from build123d import *

# Parameters (mm, degrees)
SKETCH_1_W             = 28
SKETCH_1_H             = 160
SKETCH_1_R             = 6
SKETCH_1_R_2           = 1.35
SM_BASE_FLANGE_1_DEPTH = 3
OTHER_START            = -14
OTHER_1_DEPTH          = 28
OTHER_1_2_DEPTH        = 28
SKETCH_7_R             = 1.35
CUT_EXTRUDE_1_DEPTH    = 81.582164958


# Read off the part's stored shape, not the designer's step: 绘制的折弯1
# Sheet-metal steps are written as plain solids
with BuildPart() as part:
    # Sketch 1 → 基体-法兰1 (new body)
    with BuildSketch(Plane(origin=(0, 0, 0), x_dir=(1, 0, 0), z_dir=(0, 1, 0))):
        Rectangle(SKETCH_1_W, SKETCH_1_H)
        with Locations(Location((0, 0, 0), (0, 0, 270))):
            Circle(SKETCH_1_R, mode=Mode.SUBTRACT)
        with Locations(Location((0, 11, 0), (0, 0, 270))):
            Circle(SKETCH_1_R_2, mode=Mode.SUBTRACT)
        with Locations(Location((7.778174593, 7.778174593, 0), (0, 0, 270))):
            Circle(SKETCH_1_R_2, mode=Mode.SUBTRACT)
        with Locations(Location((11, 0, 0), (0, 0, 270))):
            Circle(SKETCH_1_R_2, mode=Mode.SUBTRACT)
        with Locations(Location((7.778174593, -7.778174593, 0), (0, 0, 270))):
            Circle(SKETCH_1_R_2, mode=Mode.SUBTRACT)
        with Locations(Location((0, -11, 0), (0, 0, 270))):
            Circle(SKETCH_1_R_2, mode=Mode.SUBTRACT)
        with Locations(Location((-7.778174593, -7.778174593, 0), (0, 0, 270))):
            Circle(SKETCH_1_R_2, mode=Mode.SUBTRACT)
        with Locations(Location((-11, 0, 0), (0, 0, 270))):
            Circle(SKETCH_1_R_2, mode=Mode.SUBTRACT)
        with Locations(Location((-7.778174593, 7.778174593, 0), (0, 0, 270))):
            Circle(SKETCH_1_R_2, mode=Mode.SUBTRACT)
    extrude(amount=-SM_BASE_FLANGE_1_DEPTH)

    # Other 1 outline → Other 1 (cut)
    with BuildSketch(Plane.YZ.offset(OTHER_START)):
        with BuildLine():
            ThreePointArc((0, -31.146677222), (-2.154295979, -29.850867001), (-3, -27.4834))
            Line((-3, -27.4834), (-3, -80))
            Line((-3, -80), (0, -80))
            Line((0, -80), (0, -31.146677222))
        make_face()
        with BuildLine():
            Line((-3, 80), (-3, 22.7634))
            ThreePointArc((-3, 22.7634), (-2.154295979, 25.130867001), (0, 26.426677222))
            Line((0, 26.426677222), (0, 80))
            Line((0, 80), (-3, 80))
        make_face()
    extrude(amount=OTHER_1_DEPTH, mode=Mode.SUBTRACT)

    # Other 1 2 outline → Other 1 2 (add)
    with BuildSketch(Plane.YZ.offset(OTHER_START)):
        with BuildLine():
            Line((0, -27.4834), (0, -31.146677222))
            ThreePointArc((0, -31.146677222), (0.36647982, -31.201624121), (0.7366, -31.22))
            Line((0.7366, -31.22), (49.739956935, -31.22))
            Line((49.739956935, -31.22), (49.739956935, -28.22))
            Line((49.739956935, -28.22), (0.7366, -28.22))
            ThreePointArc((0.7366, -28.22), (0.215745145, -28.004254855), (0, -27.4834))
        make_face()
        with BuildLine():
            ThreePointArc((0.7366, 26.5), (0.36647982, 26.481624121), (0, 26.426677222))
            Line((0, 26.426677222), (0, 22.7634))
            ThreePointArc((0, 22.7634), (0.215745145, 23.284254855), (0.7366, 23.5))
            Line((0.7366, 23.5), (54.459956935, 23.5))
            Line((54.459956935, 23.5), (54.459956935, 26.5))
            Line((54.459956935, 26.5), (0.7366, 26.5))
        make_face()
    extrude(amount=OTHER_1_2_DEPTH)

    # 草图7 → 切除-拉伸1 (cut, through all)
    with BuildSketch(Plane(origin=(0, 0, -31.22), x_dir=(-1, 0, 0), z_dir=(0, 0, -1))):
        with Locations(Location((11, 32, 0), (0, 0, 90))):
            Circle(SKETCH_7_R)
        with Locations(Location((7.778174593, 24.221825407, 0), (0, 0, 90))):
            Circle(SKETCH_7_R)
        with Locations(Location((0, 21, 0), (0, 0, 90))):
            Circle(SKETCH_7_R)
        with Locations(Location((-7.778174593, 24.221825407, 0), (0, 0, 90))):
            Circle(SKETCH_7_R)
        with Locations(Location((-11, 32, 0), (0, 0, 90))):
            Circle(SKETCH_7_R)
        with BuildLine():
            Line((-14, 32), (-32.703539992, 32))
            Line((-32.703539992, 32), (-28.620805063, 56.964772816))
            Line((-28.620805063, 56.964772816), (24.538070134, 56.964772816))
            Line((24.538070134, 56.964772816), (24.538070134, 32))
            Line((24.538070134, 32), (14, 32))
            Line((14, 32), (14, 35.400052641))
            Line((14, 35.400052641), (6, 35.400052641))
            Line((6, 35.400052641), (6, 32))
            ThreePointArc((6, 32), (0, 26), (-6, 32))
            Line((-6, 32), (-6, 35.400052641))
            Line((-6, 35.400052641), (-14, 35.400052641))
            Line((-14, 35.400052641), (-14, 32))
        make_face()
    extrude(amount=-CUT_EXTRUDE_1_DEPTH, mode=Mode.SUBTRACT)


solid = part.part
Geometry check sheet. Reference: the model listing, model coordinates, mm. A direction names the side the tool comes from. Round coordinates to 2 decimals unless told otherwise and drop trailing zeros. Loops run counter-clockwise (first coordinate to the right, second up) from the corner with the lowest first, then second, coordinate; pieces in that order, holes last. Notation, with made-up numbers: (57.25, 73) - (98.25, 73) arc R11 ccw to (98.25, 83) - close; hole circle Ø5 at (-16, 77). An arc over 180 degrees is marked (long way). One line per question, with ' | ' between items. Start each with the question number.
1. Cross-section at D-D on y = 11. Record the cut outline in (x, z).
2. Tool access check on faces 1 (the face through (0, 0, -8)), 2 (the face through (6, 34, 25)), 3 (the face through (10, 35.4, 25)). Record the directions out of +Z, -Z, +X, -X, +Y, -Y that give a thin tool (end or side, any length) a straight path to the whole face; none if there is none.
3. Depth check by flat-ended pin: pin 1 (15.5 mm diameter, centred on x = 0, z = 0, fed in from +Y). Enter the tip coordinate at first touch or a pass-through.
4. Cross-section at A-A on x = 11. Record the cut outline in (y, z), then the cut area to 4 significant figures.
5. Scan lines: line 1 (X direction, y = -2.3, z = 0); line 2 (Z direction, x = 12, y = 17.5); line 3 (Y direction, x = 12.75, z = 6.5). Record each from-to range of solid material in increasing order. Write a range as [from, to].
6. Draft check along Y on faces 4 (the face through (12.138, 32.726, 24.979)), 5 (the face through (-9.862, 32.726, 24.979)), 6 (the face through (0.406, -1.479, 12.288)), 7 (the face through (-10, 35.4, 25)). Enter one of: released by +Y, released by -Y, zero draft, split by the parting line, or undercut.
7. Cross-section at B-B on y = 21. Record the cut outline in (x, z), then the cut area to 3 significant figures.
8. Cross-section at C-C on z = 0. Record the cut outline in (x, y), then the cut area to 3 significant figures.
Taken from the geometry:
1) outline: (-14, -31.22) - (14, -31.22) - (14, -28.22) - (-14, -28.22) - close; (-14, 23.5) - (14, 23.5) - (14, 26.5) - (-14, 26.5) - close
2) face 1: +X, -X, +Y | face 2: +Z, -Z, +Y | face 3: +Z, -Z, +X, -X, +Y
3) pin 1: y = 0
4) outline: (-3, -27.48) arc R3.74 ccw to (0.74, -31.22) - (30.65, -31.22) - (30.65, -28.22) - (0.74, -28.22) arc R0.74 cw to (0, -27.48) - (0, -1.35) - (-3, -1.35) - close; (-3, 1.35) - (0, 1.35) - (0, 22.76) arc R0.74 cw to (0.74, 23.5) - (30.65, 23.5) - (30.65, 26.5) - (0.74, 26.5) arc R3.74 ccw to (-3, 22.76) - close; (33.35, -31.22) - (35.4, -31.22) - (35.4, -28.22) - (33.35, -28.22) - close; (33.35, 23.5) - (35.4, 23.5) - (35.4, 26.5) - (33.35, 26.5) - close | area: 355.5 mm²
5) line 1: [-14, -12.35], [-9.65, -6], [6, 9.65], [12.35, 14] | line 2: [-31.22, -28.22], [23.5, 26.5] | line 3: [-3, 0]
6) face 4: undercut | face 5: undercut | face 6: zero draft | face 7: released by +Y
7) outline: (-14, -31.22) - (-1.35, -31.22) - (-1.35, -28.22) - (-14, -28.22) - close; (-14, 23.5) - (-1.35, 23.5) - (-1.35, 26.5) - (-14, 26.5) - close; (1.35, -31.22) - (14, -31.22) - (14, -28.22) - (1.35, -28.22) - close; (1.35, 23.5) - (14, 23.5) - (14, 26.5) - (1.35, 26.5) - close | area: 152 mm²
8) outline: (-14, -3) - (-12.35, -3) - (-12.35, 0) - (-14, 0) - close; (-9.65, -3) - (-6, -3) - (-6, 0) - (-9.65, 0) - close; (6, -3) - (9.65, -3) - (9.65, 0) - (6, 0) - close; (12.35, -3) - (14, -3) - (14, 0) - (12.35, 0) - close | area: 31.8 mm²
